```python
from build123d import *

# Parameters (mm, degrees)
SKETCH1_W           = 55.5
SKETCH1_H           = 20
BOSS_EXTRUDE1_DEPTH = 36.1
SKETCH2_W           = 7.5
SKETCH2_H           = 20
CUT_EXTRUDE1_DEPTH  = 26.6
SKETCH3_W           = 7.5
SKETCH3_H           = 20
CUT_EXTRUDE2_DEPTH  = 6
SKETCH4_R           = 2.5
BOSS_EXTRUDE2_DEPTH = 8


with BuildPart() as part:
    # Sketch1 → Boss-Extrude1 (new body)
    with BuildSketch(Plane(origin=(0, 0, 0), x_dir=(1, 0, 0), z_dir=(0, 1, 0))):
        Rectangle(SKETCH1_W, SKETCH1_H)
    extrude(amount=BOSS_EXTRUDE1_DEPTH)

    # Sketch2 → Cut-Extrude1 (cut)
    with BuildSketch(Plane.XZ):
        with Locations((24, 0)):
            Rectangle(SKETCH2_W, SKETCH2_H)
        with Locations((-24, 0)):
            Rectangle(SKETCH2_W, SKETCH2_H)
    extrude(amount=-CUT_EXTRUDE1_DEPTH, mode=Mode.SUBTRACT)

    # Sketch3 → Cut-Extrude2 (cut)
    with BuildSketch(Plane(origin=(0, 36.1, 0), x_dir=(1, 0, 0), z_dir=(0, 1, 0))):
        with Locations((24, 0)):
            Rectangle(SKETCH3_W, SKETCH3_H)
        with Locations((-24, 0)):
            Rectangle(SKETCH3_W, SKETCH3_H)
    extrude(amount=-CUT_EXTRUDE2_DEPTH, mode=Mode.SUBTRACT)

    # Sketch4 → Boss-Extrude2 (add)
    with BuildSketch(Plane(origin=(0, 36.1, 0), x_dir=(1, 0, 0), z_dir=(0, 1, 0))):
        with Locations(Location((9.85, 0, 0), (0, 0, 90))):
            Circle(SKETCH4_R)
    extrude(amount=BOSS_EXTRUDE2_DEPTH)


solid = part.part
```
Geometry: final body of the model. Coordinates: model frame, mm. A direction names the side the tool comes from. Round coordinates to 2 decimals unless told otherwise and drop trailing zeros. Loops run counter-clockwise (first coordinate to the right, second up) from the corner with the lowest first, then second, coordinate; pieces in that order, holes last.
Item 1: Reachability of faces 1 (the flat face through (20.25, 13, 0)), 2 (the flat face through (-20.25, 13, 0)), 3 (the flat face through (20.25, 33, 0)) from +Z, -Z, +X, -X, +Y, -Y: full face, straight path, thin tool, end or side. Return the list, or none.
Checked values:
face 1: +Z, -Z, +X, -Y
face 2: +Z, -Z, -X, -Y
face 3: +Z, -Z, +X, +Y
Item 2: Contact query for flat-ended pins moving along their axis: P1, Ø4, axis at x = -14, z = 5, coming from the +Y side; P2, Ø1.8, axis at y = 32.5, z = -3.5, coming from the +X side; P3, Ø6, axis at y = 21.5, z = -4.5, coming from the -X side. Output: stop coordinate, or through.
Checked values:
P1: stops at y = 36.1
P2: stops at x = 20.25
P3: stops at x = -20.25
Item 3: Line query: L1, parallel to Y at x = 15.5, z = -2.25; L2, parallel to X at y = 7.5, z = -0.5; L3, parallel to Y at x = -24.5, z = 8. Output: solid intervals per line, ascending.
Checked values:
L1: y = 0 to 36.1
L2: x = -20.25 to 20.25
L3: y = 26.6 to 30.1
Item 4: Section B-B, the plane x = 9.85. Output: boundary loops of the cut face in (y, z).
Checked values:
outline: (0, -10) - (36.1, -10) - (36.1, -2.5) - (44.1, -2.5) - (44.1, 2.5) - (36.1, 2.5) - (36.1, 10) - (0, 10) - close
Item 5: Section C-C, the plane y = 22.5. Output: boundary loops of the cut face in (x, z).
Checked values:
outline: (-20.25, -10) - (20.25, -10) - (20.25, 10) - (-20.25, 10) - close
Item 6: Section D-D, the plane z = 8.75. Output: boundary loops of the cut face in (x, y).
Checked values:
outline: (-27.75, 26.6) - (-20.25, 26.6) - (-20.25, 0) - (20.25, 0) - (20.25, 26.6) - (27.75, 26.6) - (27.75, 30.1) - (20.25, 30.1) - (20.25, 36.1) - (-20.25, 36.1) - (-20.25, 30.1) - (-27.75, 30.1) - close
Item 7: Section A-A, the plane z = 1.5. Output: boundary loops of the cut face in (x, y).
Checked values:
outline: (-27.75, 26.6) - (-20.25, 26.6) - (-20.25, 0) - (20.25, 0) - (20.25, 26.6) - (27.75, 26.6) - (27.75, 30.1) - (20.25, 30.1) - (20.25, 36.1) - (11.85, 36.1) - (11.85, 44.1) - (7.85, 44.1) - (7.85, 36.1) - (-20.25, 36.1) - (-20.25, 30.1) - (-27.75, 30.1) - close
